Source: CAD feature listing. Evaluate the final solid. Frame: model axes, mm. Face numbers are marked on the shaded views. A direction names the side the tool comes from. Coordinates: 2 decimals unless noted, no trailing zeros. Loops run counter-clockwise (first coordinate to the right, second up) from the corner with the lowest first, then second, coordinate; pieces in that order, holes last. Notation, with made-up numbers: (69.5, -38) - (86.5, -38) arc R19 cw to (86.5, -26) - close; hole circle Ø7 at (50, 63). An arc over 180 degrees is marked (long way). Use one line per item in the form item = value. Start each with the question number.
Solid Edge part; units mm, degrees
sketch "Sketch1" plane through (0, 0, 0) normal (0, 0, 1) x (1, 0, 0)
  line L0 (3, -4.75) -> (-3, -4.75)
  arc A0 (-3, 4.75) -> (-3, -4.75) centre (-3, 0) ccw
  line L1 (-3, 4.75) -> (3, 4.75)
  arc A1 (3, -4.75) -> (3, 4.75) centre (3, 0) ccw
extrude "Protrusion1" add sketch "Sketch1" against normal blind 2
sketch "Sketch2" plane through (0, 0, -2) normal (0, 0, -1) x (1, 0, 0)
  line L0 (-3.25, 2.75) -> (3.25, 2.75)
  arc A0 (3.25, -2.75) -> (3.25, 2.75) centre (3.25, 0) ccw
  line L1 (3.25, -2.75) -> (-3.25, -2.75)
  arc A1 (-3.25, 2.75) -> (-3.25, -2.75) centre (-3.25, 0) ccw
extrude "ExtrudedProtrusion_2" add sketch "Sketch2" along normal blind 8.5
sketch "Sketch3" plane through (0, 0, -10.5) normal (0, 0, -1) x (1, 0, 0)
  line L0 (-3.25, -1.25) -> (3.25, -1.25)
  arc A0 (3.25, -1.25) -> (3.25, 1.25) centre (3.25, 0) ccw
  line L1 (3.25, 1.25) -> (-3.25, 1.25)
  arc A1 (-3.25, 1.25) -> (-3.25, -1.25) centre (-3.25, 0) ccw
extrude "ExtrudedProtrusion_3" add sketch "Sketch3" along normal blind 2
sketch "Sketch4" plane through (0, 0, 0) normal (0, 0, 1) x (1, 0, 0)
  arc A0 (-3, -1.25) -> (-4, -0.25) centre (-3, -0.25) cw
  line L0 (-4, 0.25) -> (-4, -0.25)
  arc A1 (-4, 0.25) -> (-3, 1.25) centre (-3, 0.25) cw
  line L1 (3, 1.25) -> (-3, 1.25)
  arc A2 (3, 1.25) -> (4, 0.25) centre (3, 0.25) cw
  line L2 (4, -0.25) -> (4, 0.25)
  arc A3 (3, -1.25) -> (4, -0.25) centre (3, -0.25) ccw
  line L3 (-3, -1.25) -> (3, -1.25)
extrude "ExtrudedCutout_1" cut sketch "Sketch4" against normal blind 9.303
chamfer "Chamfer_1" distance 1 angle 45 4 edges at (0, 4.75, 0) (7.75, 0, 0) (0, -4.75, 0) (-7.75, 0, 0)
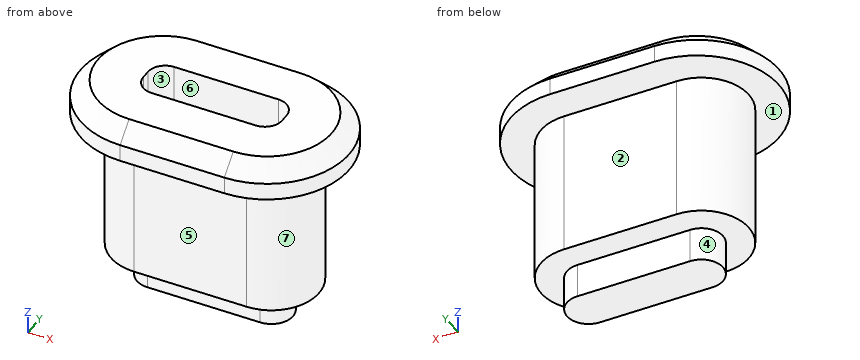
(1) Cut plane B-B, the plane y = 0. Output: boundary loops of the cut face in (x, z).
(2) Mould query, pull axis Y, two halves, no side actions, for the marked faces 1, 2 and 3. Classes: +Y half, -Y half, draft (parallel to the pull), parting line (faces both ways), or undercut.
(3) Cut plane A-A, the plane z = -5.75. Output: boundary loops of the cut face in (x, y).
(4) Contact query for flat-ended pins moving along their axis: pin 1 (7 mm diameter, centred on x = -1.5, z = -5, fed in from +Y); pin 2 (5 mm diameter, centred on x = 1.5, z = -6.5, fed in from -Y); pin 3 (5 mm diameter, centred on x = -0.5, z = -5, fed in from +Y); pin 4 (2 mm diameter, centred on x = 1.5, z = -12, fed in from -Y). Output: stop coordinate, or through.
(5) Access query for the marked faces 4, 5, 6 and 7. Directions: +Z, -Z, +X, -X, +Y, -Y. A direction counts if a zero-diameter tool reaches every point of the face in a straight line with its end or side. Return the directions, or none.
(6) Material intervals for line 1 (Y direction, x = 2.5, z = -4); line 2 (Z direction, x = 0.25, y = -2.25); line 3 (Y direction, x = 3.75, z = -5), sorted ascending.
Recorded:
q1.outline = (-7.75, -2) - (-6, -2) - (-6, -10.5) - (-4.5, -10.5) - (-4.5, -12.5) - (4.5, -12.5) - (4.5, -10.5) - (6, -10.5) - (6, -2) - (7.75, -2) - (7.75, -1) - (6.75, 0) - (4, 0) - (4, -9.3) - (-4, -9.3) - (-4, 0) - (-6.75, 0) - (-7.75, -1) - close
q2.face_1 = draft
q2.face_2 = +Y half
q2.face_3 = undercut
q3.outline = (-3.25, -2.75) - (3.25, -2.75) arc R2.75 ccw to (3.25, 2.75) - (-3.25, 2.75) arc R2.75 ccw to start; hole (-4, -0.25) arc R1 ccw to (-3, -1.25) - (3, -1.25) arc R1 ccw to (4, -0.25) - (4, 0.25) arc R1 ccw to (3, 1.25) - (-3, 1.25) arc R1 ccw to (-4, 0.25) - close
q4.pin_1 = 4.75
q4.pin_2 = -2.75
q4.pin_3 = 2.75
q4.pin_4 = -1.25
q5.face_4 = -Z, -X
q5.face_5 = -Z, +X, -X, -Y
q5.face_6 = +Z
q5.face_7 = -Z, +X
q6.line_1 = -2.75 to -1.25, 1.25 to 2.75
q6.line_2 = -10.5 to 0
q6.line_3 = -2.7 to -0.91, 0.91 to 2.7
